Drawing for the job (mm, zero at the part's lowest x, y, z). Coordinates: 2 decimals unless noted, no trailing zeros. Order: outer loops, then holes, each group sorted by start corner. A loop starts at its lowest first (then second) coordinate and runs counter-clockwise, first axis right, second up.
1) Cut at A-A (z = 54.5). List the corners of the cut face in (x, y).
2) Wall check: L1, parallel to X at y = 3, z = 4.25; L2, parallel to Y at x = 5, z = 51. Give the ranges that are in metal, low to high.
3) Pin check, flat tips, straight feed: pin 1 Ø1 at (x, y) = (5, 3) entering from -Z; pin 2 Ø1 at (x, y) = (15, 3) entering from +Z. Stop position of each tip, or through.
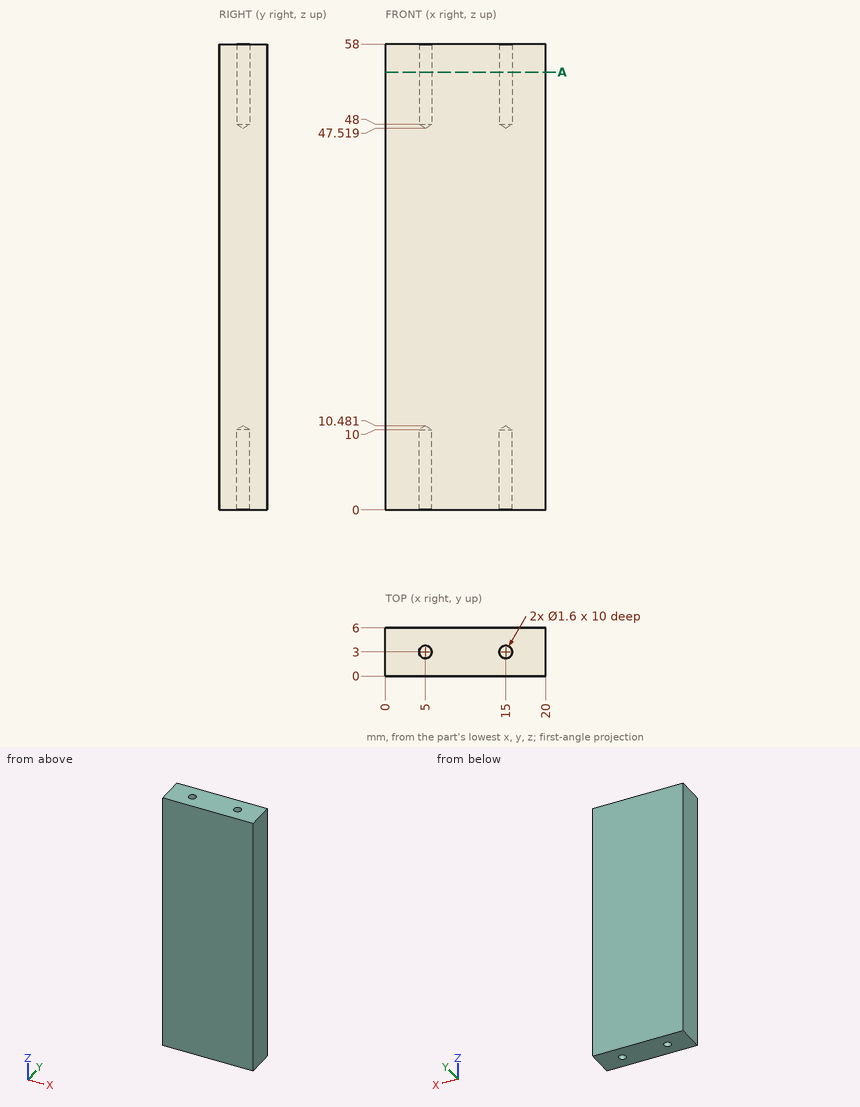
Geometry check:
1. outline: (0, 0) - (20, 0) - (20, 6) - (0, 6) - close; hole circle Ø1.6 at (5, 3); hole circle Ø1.6 at (15, 3)
2. L1: x = 0 to 4.2, 5.8 to 14.2, 15.8 to 20
2. L2: y = 0 to 2.2, 3.8 to 6
3. pin 1: stops at z = 10.18
3. pin 2: stops at z = 47.82
